```python
from build123d import *

# Parameters (mm, degrees)
SKETCH1_R           = 1.5
BOSS_EXTRUDE1_DEPTH = 6
FILLET1_R           = 20
CUT_EXTRUDE1_REACH  = 8
SKETCH5_R           = 1.25
BOSS_EXTRUDE2_DEPTH = 6
FILLET2_R           = 3
SKETCH6_W           = 6
SKETCH6_H           = 31.030846562
SKETCH6_H_2         = 27.343468982
CUT_EXTRUDE2_DEPTH  = 1
FILLET3_R           = 1.5


with BuildPart() as part:
    # Sketch1 → Boss-Extrude1 (new body)
    with BuildSketch(Plane(origin=(0, 0, 0), x_dir=(1, 0, 0), z_dir=(0, 1, 0))):
        with BuildLine():
            Line((-54.495367447, 86.395828983), (0, 60))
            Line((0, 60), (54.495367447, 86.395828983))
            ThreePointArc((54.495367447, 86.395828983), (63.474216903, 85.013506895), (65.371608634, 76.129225465))
            Line((65.371608634, 76.129225465), (40, 15))
            Line((40, 15), (65.688300647, -77.045475229))
            ThreePointArc((65.688300647, -77.045475229), (61.936793138, -86.150496915), (52.193978606, -84.717739607))
            Line((52.193978606, -84.717739607), (0, -30))
            Line((0, -30), (-52.193978606, -84.717739607))
            ThreePointArc((-52.193978606, -84.717739607), (-61.936793138, -86.150496915), (-65.688300647, -77.045475229))
            Line((-65.688300647, -77.045475229), (-40, 15))
            Line((-40, 15), (-65.371608634, 76.129225465))
            ThreePointArc((-65.371608634, 76.129225465), (-63.474216903, 85.013506895), (-54.495367447, 86.395828983))
        make_face()
        with Locations((-57.982756057, 79.195959493)):
            Circle(SKETCH1_R, mode=Mode.SUBTRACT)
        with Locations((57.982756057, 79.195959493)):
            Circle(SKETCH1_R, mode=Mode.SUBTRACT)
        with Locations((-57.982756057, -79.195959493)):
            Circle(SKETCH1_R, mode=Mode.SUBTRACT)
        with Locations((57.982756057, -79.195959493)):
            Circle(SKETCH1_R, mode=Mode.SUBTRACT)
        with Locations((-39, 65)):
            Circle(SKETCH1_R, mode=Mode.SUBTRACT)
        with Locations((39, 65)):
            Circle(SKETCH1_R, mode=Mode.SUBTRACT)
        with Locations((39, -55)):
            Circle(SKETCH1_R, mode=Mode.SUBTRACT)
        with Locations((-39, -55)):
            Circle(SKETCH1_R, mode=Mode.SUBTRACT)
    extrude(amount=BOSS_EXTRUDE1_DEPTH)

    # Fillet1
    fillet1_edges = [part.edges().sort_by_distance(p)[0] for p in [
        (0, 3, -60),
        (40, 3, -15),
        (0, 3, 30),
        (-40, 3, -15),
    ]]
    fillet(fillet1_edges, radius=FILLET1_R)

    # Sketch2 → Cut-Extrude1 (cut, up to next)
    with BuildSketch(Plane(origin=(0, 6, 0), x_dir=(1, 0, 0), z_dir=(0, 1, 0)), mode=Mode.PRIVATE) as cut_extrude1_sk1:
        with BuildLine():
            Line((-38.659149277, 58.724904233), (-26.025041931, 28.284847884))
            ThreePointArc((-26.025041931, 28.284847884), (-23.19190714, 16.020273346), (-24.520754868, 3.503060996))
            Line((-24.520754868, 3.503060996), (-37.591117294, -43.330232394))
            Line((-37.591117294, -43.330232394), (-27.496692892, -32.747707347))
            ThreePointArc((-27.496692892, -32.747707347), (0, -20.976162887), (27.496692892, -32.747707347))
            Line((27.496692892, -32.747707347), (37.591117294, -43.330232394))
            Line((37.591117294, -43.330232394), (24.520754868, 3.503060996))
            ThreePointArc((24.520754868, 3.503060996), (23.19190714, 16.020273346), (26.025041931, 28.284847884))
            Line((26.025041931, 28.284847884), (38.659149277, 58.724904233))
            Line((38.659149277, 58.724904233), (16.565095901, 48.023244958))
            ThreePointArc((16.565095901, 48.023244958), (0, 44.222625037), (-16.565095901, 48.023244958))
            Line((-16.565095901, 48.023244958), (-38.659149277, 58.724904233))
        make_face()
    cut_extrude1_tool1 = extrude(cut_extrude1_sk1.sketch, amount=-CUT_EXTRUDE1_REACH, mode=Mode.PRIVATE) & part.part
    add(cut_extrude1_tool1.solids().sort_by_distance((0, 6, -11.023996))[0], mode=Mode.SUBTRACT)

    # Sketch5 → Boss-Extrude2 (add)
    with BuildSketch(Plane(origin=(0, 6, 0), x_dir=(1, 0, 0), z_dir=(0, 1, 0))):
        with BuildLine():
            Line((-25.103227244, 1.415965109), (0, -5.589911573))
            Line((0, -5.589911573), (25.103227244, 1.415965109))
            Line((25.103227244, 1.415965109), (26.716090442, -4.363193333))
            Line((26.716090442, -4.363193333), (4, -10.702861409))
            Line((4, -10.702861409), (4, -21.187275631))
            ThreePointArc((4, -21.187275631), (0, -20.976162887), (-4, -21.187275631))
            Line((-4, -21.187275631), (-4, -10.702861409))
            Line((-4, -10.702861409), (-26.716090442, -4.363193333))
            Line((-26.716090442, -4.363193333), (-25.103227244, 1.415965109))
        make_face()
        with Locations((-10.3, -5.83)):
            Circle(SKETCH5_R, mode=Mode.SUBTRACT)
        with Locations((10.3, -5.83)):
            Circle(SKETCH5_R, mode=Mode.SUBTRACT)
    extrude(amount=-BOSS_EXTRUDE2_DEPTH)

    # Fillet2
    fillet2_edges = [part.edges().sort_by_distance(p)[0] for p in [
        (37.591117294, 3, 43.330232394),
        (-37.591117294, 3, 43.330232394),
        (38.659149277, 3, -58.724904233),
        (-38.659149277, 3, -58.724904233),
        (25.103227244, 3, -1.415965109),
        (-25.103227244, 3, -1.415965109),
        (0, 3, 5.589911573),
        (26.716090442, 3, 4.363193333),
        (4, 3, 10.702861409),
        (4, 3, 21.187275631),
        (-4, 3, 21.187275631),
        (-4, 3, 10.702861409),
        (-26.716090442, 3, 4.363193333),
    ]]
    fillet(fillet2_edges, radius=FILLET2_R)

    # Sketch6 → Cut-Extrude2 (cut)
    with BuildSketch(Plane(origin=(0, 6, 0), x_dir=(1, 0, 0), z_dir=(0, 1, 0))):
        with Locations((-39, -58.515423281)):
            Rectangle(SKETCH6_W, SKETCH6_H)
        with Locations((39, -58.515423281)):
            Rectangle(SKETCH6_W, SKETCH6_H)
        with Locations((39, 66.671734491)):
            Rectangle(SKETCH6_W, SKETCH6_H_2)
        with Locations((-39, 66.671734491)):
            Rectangle(SKETCH6_W, SKETCH6_H_2)
    extrude(amount=-CUT_EXTRUDE2_DEPTH, mode=Mode.SUBTRACT)

    # Fillet3
    fillet3_edges = [part.edges().sort_by_distance(p)[0] for p in [
        (-36, 5.5, 43),
        (-42, 5.5, 43),
        (36, 5.5, 43),
        (42, 5.5, 43),
        (36, 5.5, -53),
        (42, 5.5, -53),
        (-42, 5.5, -53),
        (-36, 5.5, -53),
    ]]
    fillet(fillet3_edges, radius=FILLET3_R)


solid = part.part
```
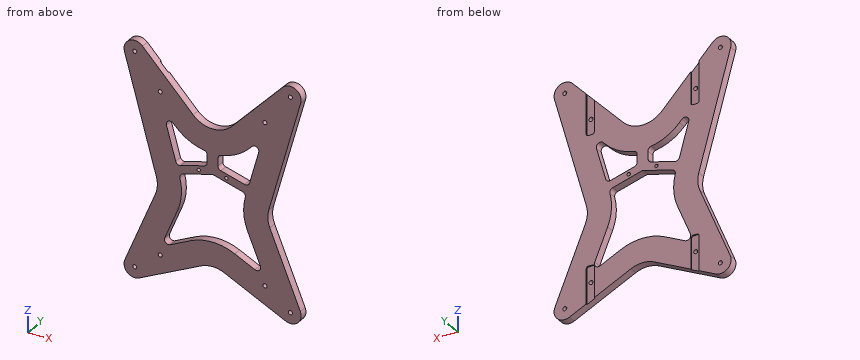
For this review, take the finished solid that the model builds, in its own axes (mm). Coordinates: 2 decimals unless noted, no trailing zeros. Loops run counter-clockwise (first coordinate to the right, second up) from the corner with the lowest first, then second, coordinate; pieces in that order, holes last.
1. For line 1 (Z direction, x = 19.5, y = 1.5); line 2 (X direction, y = 4, z = -54); line 3 (Z direction, x = -16, y = 4.5), list the stretches that pass through material, from the lowest coordinate up.
2. Add section A-A, the plane z = -34.5. Give the boundary of the cut face in (x, y), then the cut area to 3 significant figures.
3. Insertion check: P1, Ø2.5, axis at x = -39, z = 55, coming from the -Y side (1 decimal); P2, Ø1, axis at x = -28.5, y = 2, coming from the -Z side; P3, Ø2, axis at x = 5.5, y = 2.5, coming from the -Z side; P4, Ø0.5, axis at y = 5.5, z = 51, coming from the +X side. Each pin has a flat end and moves straight along its axis. Give the tip position at first contact, or say it passes through.
4. Add section D-D, the plane z = -15.5. Give the boundary of the cut face in (x, y).
5. Add section C-C, the plane y = 4. Count the separate pieces of the cut face and the enclosed holes in it, then the cut area to 3 significant figures.
6. Add section B-B, the plane z = -72.5. Give the boundary of the cut face in (x, y), then the cut area to 3 significant figures.
Result:
1. line 1: z = -69.45 to -49.44, 0.15 to 6.38, 26.36 to 50.44
1. line 2: x = -56.19 to -35.51, -28.9 to 28.9, 35.51 to 56.19
1. line 3: z = -67.75 to -47.76, 1.12 to 7.35, 24.51 to 46.77
2. outline: (-48.09, 0) - (-28.6, 0) - (-28.6, 6) - (-48.09, 6) - close; (28.6, 0) - (48.09, 0) - (48.09, 6) - (28.6, 6) - close
2. area: 234 mm2
3. P1: passes through
3. P2: stops at z = -74.05
3. P3: stops at z = -63.31
3. P4: stops at x = 58.49
4. outline: (-41.2, 0) - (-23.16, 0) - (-23.16, 6) - (-41.2, 6) - close; (23.16, 0) - (41.2, 0) - (41.2, 6) - (23.16, 6) - close
5. separate pieces: 1
5. enclosed holes: 13
5. area: 10,600 mm2
6. outline: (-63.87, 0) - (-25.81, 0) - (-25.81, 6) - (-36, 6) - (-36, 5) - (-42, 5) - (-42, 6) - (-63.87, 6) - close; (25.81, 0) - (63.87, 0) - (63.87, 6) - (42, 6) - (42, 5) - (36, 5) - (36, 6) - (25.81, 6) - close
6. area: 445 mm2
